from build123d import *

# Parameters (mm, degrees)
ESQUISSE1_W        = 149.75
ESQUISSE1_H        = 135
ESQUISSE1_R        = 1.75
BOSS_EXTRU_1_DEPTH = 3
CONG_1_R           = 5


with BuildPart() as part:
    # Esquisse1 → Boss.-Extru.1 (new body)
    with BuildSketch(Plane.XY):
        Rectangle(ESQUISSE1_W, ESQUISSE1_H)
        with Locations((-70, 62.5)):
            Circle(ESQUISSE1_R, mode=Mode.SUBTRACT)
        with Locations((70, 62.5)):
            Circle(ESQUISSE1_R, mode=Mode.SUBTRACT)
        with Locations((55, -51.5)):
            Circle(ESQUISSE1_R, mode=Mode.SUBTRACT)
        with Locations((-55, -51.5)):
            Circle(ESQUISSE1_R, mode=Mode.SUBTRACT)
        with Locations((45, 27.5)):
            Circle(ESQUISSE1_R, mode=Mode.SUBTRACT)
        with Locations((-45, 27.5)):
            Circle(ESQUISSE1_R, mode=Mode.SUBTRACT)
        with Locations((-45, -32.5)):
            Circle(ESQUISSE1_R, mode=Mode.SUBTRACT)
    extrude(amount=BOSS_EXTRU_1_DEPTH)

    # Congé1
    cong_1_edges = [part.edges().sort_by_distance(p)[0] for p in [
        (-74.875, 67.5, 1.5),
        (74.875, 67.5, 1.5),
        (74.875, -67.5, 1.5),
        (-74.875, -67.5, 1.5),
    ]]
    fillet(cong_1_edges, radius=CONG_1_R)


solid = part.part
Can you work these out from the model? Positions are in its coordinate system, mm. Coordinates: 2 decimals unless noted, no trailing zeros. Loops run counter-clockwise (first coordinate to the right, second up) from the corner with the lowest first, then second, coordinate; pieces in that order, holes last. Notation, with made-up numbers: M 76,43 L 133,43 A29 ccw 133,65 Z; hole C 21.25,-1 d4. An arc over 180 degrees is marked long. Return JSON: item names as keys, results as strings. Group by question number.
Item 1: Imagine slicing it at A-A (y = -32.5). Please give me the cut outline in (x, z) (3 decimals).
Item 2: Imagine slicing it at D-D (x = -45). Please give me the cut outline in (y, z), and give its area (3 significant figures).
Item 3: Imagine slicing it at B-B (x = 55). Please give me the cut outline in (y, z).
Item 4: I'm going to push a flat-ended pin straight in: pin 1 Ø4 at (x, y) = (-45, -32.5) entering from +Z. Where does the tip first touch, or does it pass through?
Item 5: Imagine slicing it at C-C (y = -51.5). Please give me the cut outline in (x, z) (3 decimals), and give its area (3 significant figures).
Item 6: If I drill on L1, parallel to Y at x = -45, z = 0.9; L2, parallel to Y at x = 70, z = 1.45; L3, parallel to Y at x = -55, z = 2, over which ranges is the centre line in solid material (lowest first)? Write a range as from..to.
Item 7: Thinking about a two-plate mould opening in X: for faces 1 (the cylindrical face through (71.617, 61.83, 1.479)), 2 (the cylindrical face through (46.669, 28.026, 1.479)), 3 (the flat face through (-1, 1, 3)), 4 (the cylindrical face through (-73.449, 65.996, 1.521)), which applies, released by +X, released by -X, zero draft, split by the parting line, or undercut?
Verdict:
{
 "1": {"outline": "M -74.875,0 L -46.75,0 L -46.75,3 L -74.875,3 Z; M -43.25,0 L 74.875,0 L 74.875,3 L -43.25,3 Z"},
 "2": {"outline": "M -67.5,0 L -34.25,0 L -34.25,3 L -67.5,3 Z; M -30.75,0 L 25.75,0 L 25.75,3 L -30.75,3 Z; M 29.25,0 L 67.5,0 L 67.5,3 L 29.25,3 Z", "area": "384 mm^2"},
 "3": {"outline": "M -67.5,0 L -53.25,0 L -53.25,3 L -67.5,3 Z; M -49.75,0 L 67.5,0 L 67.5,3 L -49.75,3 Z"},
 "4": {"pin 1": "stops at z = 3"},
 "5": {"outline": "M -74.875,0 L -56.75,0 L -56.75,3 L -74.875,3 Z; M -53.25,0 L 53.25,0 L 53.25,3 L -53.25,3 Z; M 56.75,0 L 74.875,0 L 74.875,3 L 56.75,3 Z", "area": "428 mm^2"},
 "6": {"L1": "y = -67.5..-34.25, -30.75..25.75, 29.25..67.5", "L2": "y = -67.5..60.75, 64.25..67.5", "L3": "y = -67.5..-53.25, -49.75..67.5"},
 "7": {"face 1": "undercut", "face 2": "undercut", "face 3": "zero draft", "face 4": "released by -X"}
}
